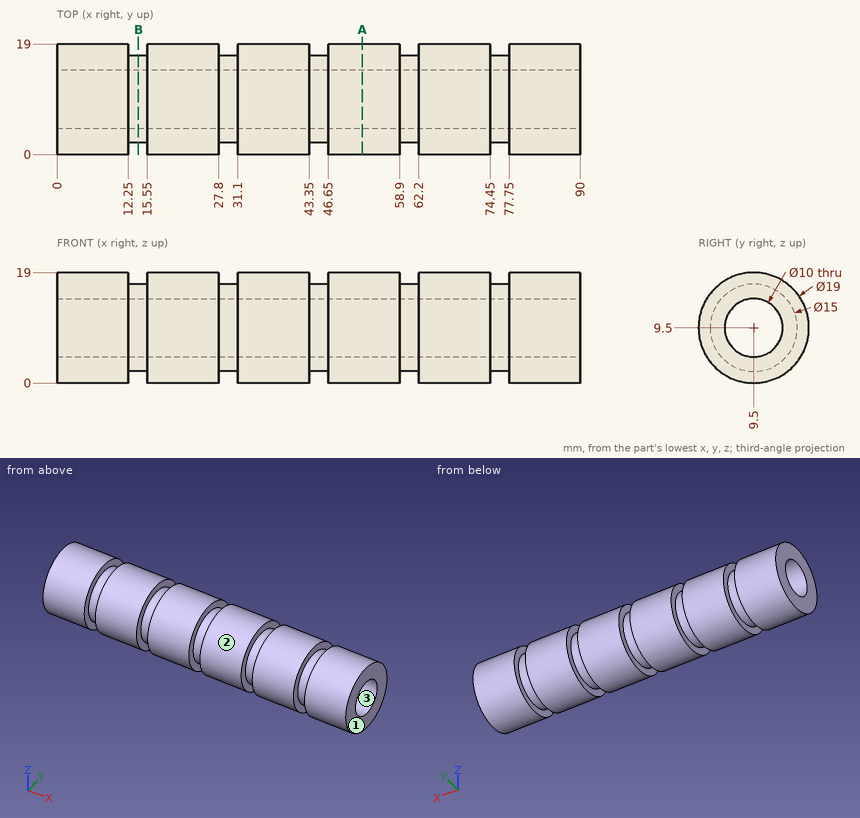
Design review of the part shown in the three views and the two pictorial views. Dimensions are in mm from the part's minimum x, y and z. Round coordinates to 2 decimals unless told otherwise and drop trailing zeros. Loops run counter-clockwise (first coordinate to the right, second up) from the corner with the lowest first, then second, coordinate; pieces in that order, holes last.
1) Wall thickness on line 1 along X through (y, z) = (17.25, 8); line 2 along Z through (x, y) = (60.5, 9.5); line 3 along Z through (x, y) = (21, 9.5): over which ranges is each line inside the solid? List them lowest first.
Values follow:
line 1: x = 0 to 12.25, 15.55 to 27.8, 31.1 to 43.35, 46.65 to 58.9, 62.2 to 74.45, 77.75 to 90
line 2: z = 2 to 4.5, 14.5 to 17
line 3: z = 0 to 4.5, 14.5 to 19
2) Consider section B-B on x = 14. State the section outline as (y, z) points, then the cut area to 3 significant figures.
Values follow:
outline: circle Ø15 at (9.5, 9.5); hole circle Ø10 at (9.5, 9.5)
area: 98.2 mm2
3) Clearance check with flat-ended pins moving along their axes: P1, Ø1, axis at x = 65.5, y = 12, coming from the +Z side; P2, Ø2, axis at x = 64, y = 14, coming from the +Z side; P3, Ø5, axis at x = 71, y = 4.5, coming from the +Z side. State where each tip first meets the part, or that it passes through.
Values follow:
P1: stops at z = 18.79
P2: stops at z = 18.33
P3: stops at z = 18.67
4) Consider section A-A on x = 52.5. State the section outline as (y, z) points.
Values follow:
outline: circle Ø19 at (9.5, 9.5); hole circle Ø10 at (9.5, 9.5)
5) The part is to be moulded in two halves that separate along Z. For the marked faces 1, 2 and 3, say which applies: pulls with the +Z half, pulls with the -Z half, needs draft (parallel to the pull), parting line crosses it, or undercut.
Values follow:
face 1: needs draft
face 2: parting line crosses it
face 3: undercut
